Autodesk Inventor part; units mm, degrees
ref_plane "YZ Plane" through (0, 0, 0) normal (1, 0, 0) x (0, 1, 0)
ref_plane "XZ Plane" through (0, 0, 0) normal (0, 1, 0) x (-1, 0, 0)
ref_plane "XY Plane" through (0, 0, 0) normal (0, 0, 1) x (1, 0, 0)
sketch "Sketch1" plane through (0, 0, 0) normal (0, 1, 0) x (-1, 0, 0)
  line L0 (0, 0) -> (-50, 0)
  line L1 (-50, 0) -> (-50, -100)
  line L2 (-50, -100) -> (0, -100)
  line L3 (0, -100) -> (0, 0)
  dimension "d0" = 100
  dimension "d1" = 50
extrude "Base" add sketch "Sketch1" along normal blind 3
sketch "Sketch2" plane through (0, 3, 0) normal (0, 1, 0) x (1, 0, 0)
  line L0 (0, 0) -> (50, 0)
  line L1 (50, 100) -> (0, 100)
  line L2 (0, 0) -> (3, 0)
  line L3 (3, 100) -> (0, 100)
  line L4 (0, 100) -> (0, 0)
  line L5 (0, 100) -> (0, 0)
  line L6 (0, 0) -> (3, 0)
  line L7 (3, 0) -> (3, 15)
  line L8 (3, 15) -> (0, 15)
  line L9 (0, 15) -> (0, 0)
  line L10 (0, 100) -> (3, 100)
  line L11 (3, 100) -> (3, 85)
  line L12 (3, 85) -> (0, 85)
  line L13 (0, 85) -> (0, 100)
  line L14 (0, 35) -> (3, 35)
  line L15 (3, 35) -> (3, 65)
  line L16 (3, 65) -> (0, 65)
  line L17 (0, 65) -> (0, 35)
  line L18 (25, 0) -> (25, 100) construction
  line L19 (50, 0) -> (47, 0)
  line L20 (47, 100) -> (50, 100)
  line L21 (50, 100) -> (50, 0)
  line L22 (50, 100) -> (50, 0)
  line L23 (50, 0) -> (47, 0)
  line L24 (47, 0) -> (47, 15)
  line L25 (47, 15) -> (50, 15)
  line L26 (50, 15) -> (50, 0)
  line L27 (50, 100) -> (47, 100)
  line L28 (47, 100) -> (47, 85)
  line L29 (47, 85) -> (50, 85)
  line L30 (50, 85) -> (50, 100)
  line L31 (50, 35) -> (47, 35)
  line L32 (47, 35) -> (47, 65)
  line L33 (47, 65) -> (50, 65)
  line L34 (50, 65) -> (50, 35)
  line L35 (0, 50) -> (50, 50) construction
  line L36 (50, 0) -> (50, 100)
  line L37 (15, 0) -> (3, 0)
  line L38 (3, 0) -> (3, 3)
  line L39 (3, 3) -> (15, 3)
  line L40 (15, 3) -> (15, 0)
  line L41 (50, 0) -> (0, 0)
  line L42 (35, 0) -> (47, 0)
  line L43 (47, 3) -> (35, 3)
  line L44 (35, 3) -> (35, 0)
  line L45 (0, 100) -> (50, 100)
  line L46 (25, 100) -> (25, 0) construction
  line L47 (15, 100) -> (3, 100)
  line L48 (3, 97) -> (15, 97)
  line L49 (15, 97) -> (15, 100)
  line L50 (50, 100) -> (0, 100)
  line L51 (47, 97) -> (35, 97)
  line L52 (35, 100) -> (47, 100)
  line L53 (35, 97) -> (35, 100)
  point P0 (0, 15)
  point P1 (0, 85)
  point P2 (3, 100)
  point P3 (0, 100)
  point P4 (0, 65)
  point P5 (0, 35)
  point P6 (47, 100)
  point P7 (50, 100)
  point P8 (47, 97)
  point P9 (35, 100)
  point P10 (15, 100)
  point P11 (3, 97)
  dimension "d10" = 15
  dimension "d11" = 15
  dimension "d12" = 20
  dimension "d13" = 20
  dimension "d14" = 30
  dimension "d15" = 3
  dimension "d21" = 3
  dimension "d22" = 10
extrude "Tabs" cut sketch "Sketch2" against normal through all contours L4 L8 L7 L0 | L7 L39 L40 L0 | L4 L16 L15 L14 | L44 L43 L24 L0 | L24 L25 L21 L0 | L4 L1 L11 L12 | L1 L49 L48 L11 | L31 L32 L33 L21 | L1 L28 L51 L53 | L29 L28 L1 L21
equation "\"d0\" = Width"
equation "\"d10\" = WidthTabOffset"
equation "\"d11\" = d10"
equation "\"d12\" = BaseTabWidth"
equation "\"d13\" = d12"
equation "\"d15\" = Thickness"
equation "\"d21\" = d15"
equation "\"d22\" = 0.5 * BaseTabWidth"
properties part number "ShortSide"
Check sheet for the modelled part. Datum: model origin and axes. Units: mm. A direction names the side the tool comes from. Round coordinates to 2 decimals unless told otherwise and drop trailing zeros. Order: outer loops, then holes, each group sorted by start corner. A loop starts at its lowest first (then second) coordinate and runs counter-clockwise, first axis right, second up.
1) Tool access check on faces 4 (the flat face through (3, 2, -9)), 5 (the flat face through (15, 2, -98)), 6 (the flat face through (2, 2, -65)), 7 (the flat face through (47, 2, -9)), 8 (the flat face through (49, 2, -35)). Record the directions out of +Z, -Z, +X, -X, +Y, -Y that give a thin tool (end or side, any length) a straight path to the whole face; none if there is none.
2) Mould release check, pull along Z, two halves, no side actions. Record for faces 1 (the flat face through (48, 2, -65)), 2 (the flat face through (50, 1, -25)), 3 (the flat face through (48, 2, -85)): +Z half, -Z half, draft (parallel to the pull), parting line (faces both ways), or undercut.
3) Scan lines: line 1 (X direction, y = 2.2, z = -11.5); line 2 (Z direction, x = 4.5, y = 2.05). Record each from-to range of solid material in increasing order.
4) Go/stop test with flat-tipped pins: pin 1 Ø8 at (x, z) = (44, -23.5) entering from -Y; pin 2 Ø1.5 at (y, z) = (2, -52) entering from +X; pin 3 Ø0.9 at (x, y) = (1.5, 2) entering from -Z; pin 4 Ø1.5 at (x, y) = (43, 1.5) entering from -Z. Record where each tip stops, or that it passes through.
5) Section check A-A (y = 2.55). Record the boundary of the cut face in (x, z).
6) Section check C-C (z = -51.5). Record the boundary of the cut face in (x, y).
7) Section check B-B (x = 12). Record the boundary of the cut face in (y, z).
Result:
1. face 4: +Z, -X, +Y, -Y
1. face 5: -Z, -X, +Y, -Y
1. face 6: -X, +Y, -Y
1. face 7: +Z, +X, +Y, -Y
1. face 8: +X, +Y, -Y
2. face 1: undercut
2. face 2: draft
2. face 3: -Z half
3. line 1: x = 3 to 47
3. line 2: z = -97 to -3
4. pin 1: stops at y = 0
4. pin 2: stops at x = 47
4. pin 3: stops at z = -85
4. pin 4: stops at z = -97
5. outline: (0, -85) - (3, -85) - (3, -97) - (15, -97) - (15, -100) - (35, -100) - (35, -97) - (47, -97) - (47, -85) - (50, -85) - (50, -65) - (47, -65) - (47, -35) - (50, -35) - (50, -15) - (47, -15) - (47, -3) - (35, -3) - (35, 0) - (15, 0) - (15, -3) - (3, -3) - (3, -15) - (0, -15) - (0, -35) - (3, -35) - (3, -65) - (0, -65) - close
6. outline: (3, 0) - (47, 0) - (47, 3) - (3, 3) - close
7. outline: (0, -97) - (3, -97) - (3, -3) - (0, -3) - close
